from build123d import *

# Parameters (mm, degrees)
SKIZZE2_R = 10


with BuildPart() as part:
    # Austragung1: sweep along a path in Skizze1
    with BuildLine(Plane.XY) as austragung1_path:
        Line((25, 300), (-5, 300))
        ThreePointArc((-5, 300), (-19.142135624, 294.142135624), (-25, 280))
        Line((-25, 280), (-25, -280))
        ThreePointArc((-25, -280), (-19.142135624, -294.142135624), (-5, -300))
        Line((-5, -300), (25, -300))
    # Skizze2 → Austragung1 (sweep)
    with BuildSketch(Plane(origin=(25, 0, 0), x_dir=(0, 0, -1), z_dir=(1, 0, 0))):
        with Locations((0, 300)):
            Circle(SKIZZE2_R)
    sweep(path=austragung1_path.line)


solid = part.part
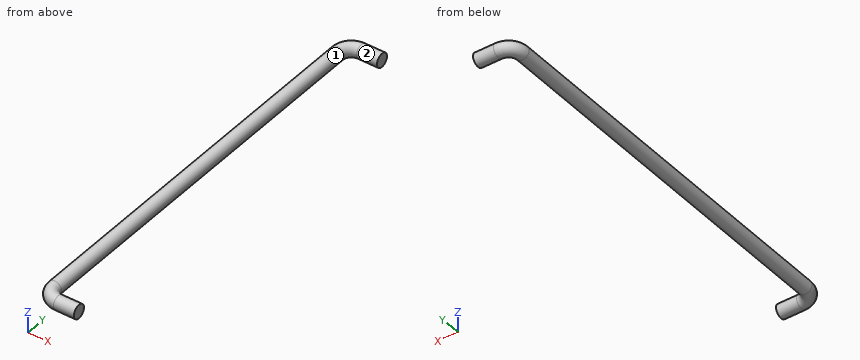
The model under review builds one solid part; all positions refer to its coordinate system, in mm. Face numbers are marked on the shaded views. A direction names the side the tool comes from. Coordinates: 2 decimals unless noted, no trailing zeros. Order: outer loops, then holes, each group sorted by start corner. A loop starts at its lowest first (then second) coordinate and runs counter-clockwise, first axis right, second up. Notation, with made-up numbers: (-12.5, -13.75) -> (6.5, -13.75) arc R27 ccw to (6.5, 9.25) -> close; hole circle Ø11 at (64, 43.25). An arc over 180 degrees is marked (long way). Answer in a Markdown table with one row per item.
(1) Wall thickness on line 1 along Y through (x, z) = (13, 7.5); line 2 along Y through (x, z) = (14, -1); line 3 along X through (y, z) = (-23, 0): over which ranges is each line inside the solid? List them lowest first.
Answers:
| item | result |
|---|---|
| line 1 | -306.61 to -293.39, 293.39 to 306.61 |
| line 2 | -309.95 to -290.05, 290.05 to 309.95 |
| line 3 | -35 to -15 |
(2) Insertion check: pin 1 (12 mm diameter, centred on x = -22.5, z = -7, fed in from -Y); pin 2 (1 mm diameter, centred on y = -90.5, z = 7.5, fed in from -X); pin 3 (6 mm diameter, centred on x = 9, z = -6, fed in from -Y). Each pin has a flat end and moves straight along its axis. Give the tip position at first contact, or say it passes through.
Answers:
| item | result |
|---|---|
| pin 1 | y = -306.52 |
| pin 2 | x = -32.14 |
| pin 3 | y = -309.54 |
(3) Consider section B-B (x = 18). Write out the cut boundary in (y, z).
Answers:
| item | result |
|---|---|
| outline | circle Ø20 at (-300, 0); circle Ø20 at (300, 0) |
(4) Machinability: for the marked faces 1 and 2, which of the approach directions +Z, -Z, +X, -X, +Y, -Y give a long, thin tool a straight path to every point of the face, cutting with its end or side? Answer none if there is none.
Answers:
| item | result |
|---|---|
| face 1 | none |
| face 2 | +X |
(5) Consider section A-A (z = 0). Write out the cut boundary in (x, y).
Answers:
| item | result |
|---|---|
| outline | (-35, -280) arc R30 ccw to (-5, -310) -> (25, -310) -> (25, -290) -> (-5, -290) arc R10 cw to (-15, -280) -> (-15, 280) arc R10 cw to (-5, 290) -> (25, 290) -> (25, 310) -> (-5, 310) arc R30 ccw to (-35, 280) -> close |
(6) Consider section C-C (y = -201.5). Write out the cut boundary in (x, z).
Answers:
| item | result |
|---|---|
| outline | circle Ø20 at (-25, 0) |
